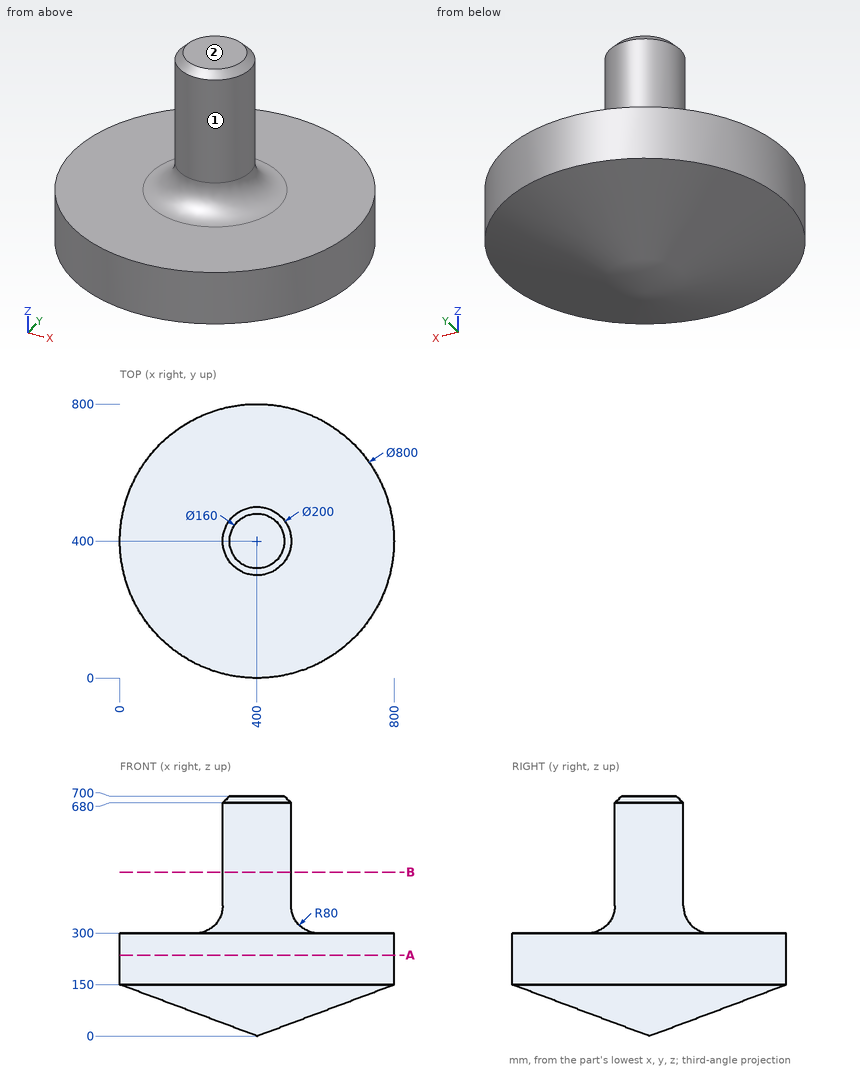
Design review of the part shown in the three views and the two pictorial views. Dimensions are in mm from the part's minimum x, y and z. A direction names the side the tool comes from. Give positions to 0.01 mm unless a question says otherwise; leave off trailing zeros. Write each loop counter-clockwise with the first axis right and the second up, starting at its lowest first coordinate (ties: lowest second). Pieces come first, ordered by that corner, then holes. Notation, with made-up numbers: M 15.5,6.25 L 28.5,6.25 A16 ccw 28.5,27.25 Z; hole C -35,25 d11. An arc over 180 degrees is marked long. One line per question, with ' | ' between items. Start each with the question number.
Item 1: We need section B-B on z = 478.5. Write out the cut boundary in (x, y).
Item 2: Wall thickness on line 1 (X direction, y = 127, z = 266); line 2 (Z direction, x = 252.5, y = 547.5); line 3 (Y direction, x = 327.5, z = 317.5): over which ranges is each line inside the solid? List them lowest first. Write a range as from..to.
Item 3: For pin 1 (5 mm diameter, centred on x = 484, y = 396, fed in from -Z); pin 2 (8 mm diameter, centred on x = 488, z = 461, fed in from -Y); pin 3 (1 mm diameter, centred on y = 434, z = 243.5, fed in from +X), all flat-tipped, find the tip position at first contact; note any pin that passes through.
Item 4: For the marked faces 1 and 2, list the 3-axis set-ups (+Z, -Z, +X, -X, +Y, -Y) from which the entire face can be reached by the end or side of a thin tool; tool diameter is ignored.
Item 5: We need section A-A on z = 236. Write out the cut boundary in (x, y).
Results found:
1) outline: C 400,400 d200
2) line 1: x = 107.65..692.35 | line 2: z = 78.22..300 | line 3: y = 292.02..507.98
3) pin 1: stops at z = 30.6 | pin 2: stops at y = 345.74 | pin 3: stops at x = 798.59
4) face 1: +Z | face 2: +Z, +X, -X, +Y, -Y
5) outline: C 400,400 d800
